```python
from build123d import *

# Parameters (mm, degrees)
F0_W     = 70
F0_H     = 70
F1_DEPTH = 60
F2_W     = 40
F2_H     = 50
F3_DEPTH = 50
F4_W     = 20
F4_H     = 40
F5_DEPTH = 20
F6_W     = 40
F6_H     = 40
F7_DEPTH = 30
F8_R     = 20
F9_SIZE  = 10


with BuildPart() as f1:
    # F0 (on Top) → F1 (new body)
    with BuildSketch(Plane.XY):
        with Locations((35, 35)):
            Rectangle(F0_W, F0_H)
    extrude(amount=F1_DEPTH)

    # F2 (on face) → F3 (cut)
    with BuildSketch(Plane.XY.offset(60)):
        with Locations((50, 25)):
            Rectangle(F2_W, F2_H)
    extrude(amount=-F3_DEPTH, mode=Mode.SUBTRACT)

    # F4 (on face) → F5 (cut)
    with BuildSketch(Plane.XZ.offset(-50)):
        with Locations((60, 40)):
            Rectangle(F4_W, F4_H)
    extrude(amount=-F5_DEPTH, mode=Mode.SUBTRACT)

    # F6 (on face) → F7 (cut)
    with BuildSketch(Plane.YZ.offset(30)):
        with Locations((20, 40)):
            Rectangle(F6_W, F6_H)
    extrude(amount=-F7_DEPTH, mode=Mode.SUBTRACT)

    # F8
    f8_edges = [f1.edges().sort_by_distance(p)[0] for p in [
        (15, 40, 20),
    ]]
    fillet(f8_edges, radius=F8_R)

    # F9
    f9_edges = [f1.edges().sort_by_distance(p)[0] for p in [
        (50, 50, 10),
    ]]
    chamfer(f9_edges, length=F9_SIZE)


solid = f1.part
```
Check sheet for the modelled part. Datum: model origin and axes. Units: mm. A direction names the side the tool comes from. Round coordinates to 2 decimals unless told otherwise and drop trailing zeros. Write each loop counter-clockwise with the first axis right and the second up, starting at its lowest first coordinate (ties: lowest second). Pieces come first, ordered by that corner, then holes. Notation, with made-up numbers: (7.25, 60.25) -> (43.25, 60.25) arc R20 ccw to (43.25, 94.25) -> close; hole circle Ø9 at (-17, 10). An arc over 180 degrees is marked (long way). One line per question, with ' | ' between items. Start each with the question number.
1. Sectioned sample at B-B, the plane x = 15. Record the cut outline in (y, z).
2. Sectioned sample at A-A, the plane z = 28. Record the cut outline in (x, y).
3. Scan lines: line 1 along Y through (x, z) = (8, 54); line 2 along X through (y, z) = (54, 50.5); line 3 along X through (y, z) = (45.5, 23). Record each from-to range of solid material in increasing order. Write a range as from..to.
4. Sectioned sample at D-D, the plane x = 38. Record the cut outline in (y, z), then the cut area to 3 significant figures.
5. Depth check by flat-ended pin: pin 1 (6 mm diameter, centred on y = 46, z = 31.5, fed in from +X); pin 2 (22 mm diameter, centred on x = 64.5, y = 58.5, fed in from +Z); pin 3 (1 mm diameter, centred on x = 14.5, z = 39, fed in from -Y). Enter the tip coordinate at first touch or a pass-through.
6. Set-up check for faces 1 (the face through (50, 45, 15)), 2 (the face through (50, 60, 40)), 3 (the face through (15, 10, 20)): record each of +Z, -Z, +X, -X, +Y, -Y from which the full face is reachable in a straight line by a thin tool's end or side.
7. Sectioned sample at C-C, the plane y = 52. Record the cut outline in (x, z), then the cut area to 3 significant figures.
Taken from the geometry:
1) outline: (0, 0) -> (70, 0) -> (70, 60) -> (40, 60) -> (40, 40) arc R20 cw to (20, 20) -> (0, 20) -> close
2) outline: (0, 36) -> (30, 36) -> (30, 50) -> (50, 50) -> (50, 70) -> (0, 70) -> close
3) line 1: y = 40..70 | line 2: x = 0..50 | line 3: x = 0..30
4) outline: (0, 0) -> (70, 0) -> (70, 60) -> (50, 60) -> (50, 20) -> (40, 10) -> (0, 10) -> close | area: 1,750 mm^2
5) pin 1: stops at x = 30 | pin 2: stops at z = 20 | pin 3: stops at y = 39.94
6) face 1: +Z, +X, -Y | face 2: +Z, +X, +Y, -Y | face 3: +Z, +X, -X, -Y
7) outline: (0, 0) -> (70, 0) -> (70, 20) -> (50, 20) -> (50, 60) -> (0, 60) -> close | area: 3,400 mm^2
